Build history of the part. All positions in model axes, mm. Face numbers are marked on the shaded views. A direction names the side the tool comes from. Round coordinates to 2 decimals unless told otherwise and drop trailing zeros. Write each loop counter-clockwise with the first axis right and the second up, starting at its lowest first coordinate (ties: lowest second). Pieces come first, ordered by that corner, then holes. Notation, with made-up numbers: (64, 81.5) -> (88, 81.5) arc R17 cw to (88, 96.5) -> close; hole circle Ø10 at (-21, -14.5). An arc over 180 degrees is marked (long way). Return JSON: item names as keys, results as strings.
from build123d import *

# Parameters (mm, degrees)
F0_R     = 12.192
F0_R_2   = 9.3345
F1_DEPTH = 3.4925
F2_DEPTH = 12.7
F0_R_3   = 38.1
F3_DEPTH = 3.4925


with BuildPart() as f1:
    # F0 (on Top) → F1 (new body)
    with BuildSketch(Plane.XY):
        Circle(F0_R)
        Circle(F0_R_2, mode=Mode.SUBTRACT)
    extrude(amount=F1_DEPTH)

    # F0 (on Top) → F2 (join)
    with BuildSketch(Plane.XY):
        Circle(F0_R_2)
    extrude(amount=F2_DEPTH)

    # F0 (on Top) → F3 (join)
    with BuildSketch(Plane.XY):
        Circle(F0_R_3)
        Circle(F0_R, mode=Mode.SUBTRACT)
        Circle(F0_R)
        Circle(F0_R_2, mode=Mode.SUBTRACT)
        Circle(F0_R_2)
    extrude(amount=-F3_DEPTH)


solid = f1.part
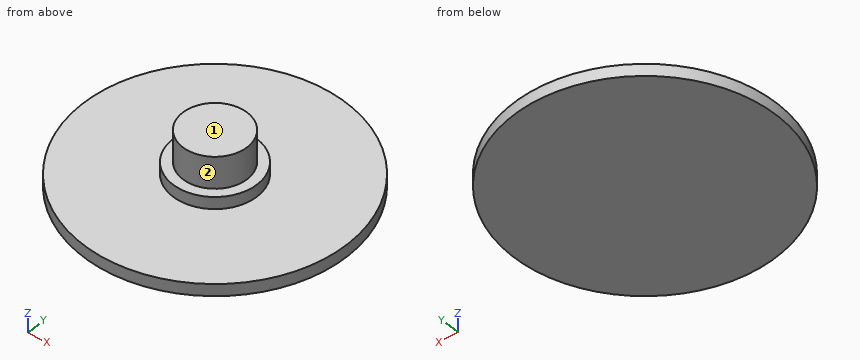
Q1. Saw through at C-C on z = 8.5. List the corners of the cut face in (x, y), then the cut area to 3 significant figures.
Verdict:
{"outline": "circle Ø18.67 at (0, 0)", "area": "274 mm²"}
Q2. Pin check, flat tips, straight feed: pin 1 Ø3 at (x, y) = (-23, -25.5) entering from +Z; pin 2 Ø4 at (y, z) = (20, -2) entering from -X; pin 3 Ø3 at (x, y) = (9, -9.5) entering from +Z. Stop position of each tip, or through.
Verdict:
{"pin 1": "stops at z = 0", "pin 2": "stops at x = -33.58", "pin 3": "stops at z = 3.49"}
Q3. 3-axis set-ups, long thin cutter, end or side, ignore diameter. For the marked faces 1 and 2: which of +Z, -Z, +X, -X, +Y, -Y reach the whole face in a straight line?
Verdict:
{"face 1": "+Z, +X, -X, +Y, -Y", "face 2": "+Z"}
Q4. Saw through at A-A on y = 0. List the corners of the cut face in (x, z).
Verdict:
{"outline": "(-38.1, -3.49) -> (38.1, -3.49) -> (38.1, 0) -> (12.19, 0) -> (12.19, 3.49) -> (9.33, 3.49) -> (9.33, 12.7) -> (-9.33, 12.7) -> (-9.33, 3.49) -> (-12.19, 3.49) -> (-12.19, 0) -> (-38.1, 0) -> close"}
Q5. Saw through at D-D on z = -1.75. List the corners of the cut face in (x, y), then the cut area to 3 significant figures.
Verdict:
{"outline": "circle Ø76.2 at (0, 0)", "area": "4,560 mm²"}
Q6. Wall check: L1, parallel to Z at x = -14, y = 13.5; L2, parallel to Z at x = -2.5, y = -10.5; L3, parallel to X at y = -6, z = 4.5. Give the ranges that are in metal, low to high.
Verdict:
{"L1": "z = -3.49 to 0", "L2": "z = -3.49 to 3.49", "L3": "x = -7.15 to 7.15"}
